from build123d import *

# Parameters (mm, degrees)
CROQUIS1_R              = 2.5
SALIENTE_EXTRUIR1_DEPTH = 5
REDONDEO1_R             = 0.5
REDONDEO2_R             = 0.2


with BuildPart() as part:
    # Croquis1 → Saliente-Extruir1 (new body)
    with BuildSketch(Plane(origin=(0, 0, 0), x_dir=(1, 0, 0), z_dir=(0, 1, 0))):
        Polygon((-2.886751346, 5), (-5.773502692, 0), (-2.886751346, -5), (2.886751346, -5), (5.773502692, 0), (2.886751346, 5), align=None)
        with Locations(Location((0, 0, 0), (0, 0, 270))):
            Circle(CROQUIS1_R, mode=Mode.SUBTRACT)
    extrude(amount=SALIENTE_EXTRUIR1_DEPTH)

    # Redondeo1
    redondeo1_edges = [part.edges().sort_by_distance(p)[0] for p in [
        (2.886751346, 2.5, -5),
        (5.773502692, 2.5, 0),
        (2.886751346, 2.5, 5),
        (-2.886751346, 2.5, 5),
        (-5.773502692, 2.5, 0),
        (-2.886751346, 2.5, -5),
    ]]
    fillet(redondeo1_edges, radius=REDONDEO1_R)

    # Redondeo2
    redondeo2_edges = [part.edges().sort_by_distance(p)[0] for p in [
        (-4.330127019, 0, -2.5),
        (-4.330127019, 5, -2.5),
        (0, 0, -5),
        (4.330127019, 0, -2.5),
        (4.330127019, 0, 2.5),
        (0, 0, 5),
        (-4.330127019, 0, 2.5),
        (-2.848076211, 0, 4.933012702),
        (-5.696152423, 0, 0),
        (2.848076211, 0, 4.933012702),
        (5.696152423, 0, 0),
        (2.848076211, 0, -4.933012702),
        (-2.848076211, 0, -4.933012702),
        (0, 5, -5),
        (-4.330127019, 5, 2.5),
        (0, 5, 5),
        (4.330127019, 5, 2.5),
        (4.330127019, 5, -2.5),
        (-2.848076211, 5, 4.933012702),
        (-5.696152423, 5, 0),
        (2.848076211, 5, 4.933012702),
        (5.696152423, 5, 0),
        (2.848076211, 5, -4.933012702),
        (-2.848076211, 5, -4.933012702),
    ]]
    fillet(redondeo2_edges, radius=REDONDEO2_R)


solid = part.part
Design review of the part built by this model. Coordinates are the model's own, in mm. Coordinates: 2 decimals unless noted, no trailing zeros. Order: outer loops, then holes, each group sorted by start corner. A loop starts at its lowest first (then second) coordinate and runs counter-clockwise, first axis right, second up.
Item 1: For pin 1 Ø1 at (y, z) = (2, -3) entering from -X, flat-tipped, find the tip position at first contact; note if it passes through.
Item 2: Take a section at C-C, the plane y = 2.7. Write out the cut boundary in (x, z).
Item 3: Take a section at B-B, the plane z = 0. Write out the cut boundary in (x, y).
Item 4: Take a section at A-A, the plane x = 0. Write out the cut boundary in (y, z), then the cut area to 3 significant figures.
Item 5: The part is to be moulded in two halves that separate along Z. For faces 1 (the flat face through (4.348, 2.468, -2.469)), 2 (the flat face through (-3, 5, 0)), 3 (the cylindrical face through (-2.44, 2.46, -0.54)), say which applies: pulls with the +Z half, pulls with the -Z half, needs draft (parallel to the pull), parting line crosses it, or undercut.
Item 6: For line 1 (X direction, y = 3.5, z = 0); line 2 (Z direction, x = 1.5, y = 1.3); line 3 (Z direction, x = -1, y = 3.8), list the stretches that pass through material, from the lowest coordinate up.
The answers:
1. pin 1: stops at x = -4.33
2. outline: (-5.63, -0.25) - (-3.03, -4.75) arc R0.5 ccw to (-2.6, -5) - (2.6, -5) arc R0.5 ccw to (3.03, -4.75) - (5.63, -0.25) arc R0.5 ccw to (5.63, 0.25) - (3.03, 4.75) arc R0.5 ccw to (2.6, 5) - (-2.6, 5) arc R0.5 ccw to (-3.03, 4.75) - (-5.63, 0.25) arc R0.5 ccw to start; hole circle Ø5 at (0, 0)
3. outline: (-5.7, 0.2) arc R0.2 ccw to (-5.5, 0) - (-2.5, 0) - (-2.5, 5) - (-5.5, 5) arc R0.2 ccw to (-5.7, 4.8) - close; (2.5, 0) - (5.5, 0) arc R0.2 ccw to (5.7, 0.2) - (5.7, 4.8) arc R0.2 ccw to (5.5, 5) - (2.5, 5) - close
4. outline: (0, -4.8) arc R0.2 ccw to (0.2, -5) - (4.8, -5) arc R0.2 ccw to (5, -4.8) - (5, -2.5) - (0, -2.5) - close; (0, 2.5) - (5, 2.5) - (5, 4.8) arc R0.2 ccw to (4.8, 5) - (0.2, 5) arc R0.2 ccw to (0, 4.8) - close
4. area: 25.0 mm2
5. face 1: pulls with the -Z half
5. face 2: needs draft
5. face 3: undercut
6. line 1: x = -5.7 to -2.5, 2.5 to 5.7
6. line 2: z = -5 to -2, 2 to 5
6. line 3: z = -5 to -2.29, 2.29 to 5
